Build history of the part. All positions in model axes, mm. A direction names the side the tool comes from. Round coordinates to 2 decimals unless told otherwise and drop trailing zeros. Write each loop counter-clockwise with the first axis right and the second up, starting at its lowest first coordinate (ties: lowest second). Pieces come first, ordered by that corner, then holes. Notation, with made-up numbers: (-29, 32.25) - (-1, 32.25) arc R15 cw to (-1, 60.25) - close; hole circle Ø8 at (-10.75, 44). An arc over 180 degrees is marked (long way). Answer as a JSON object with one key per item and string values. Group by question number.
Item 1: Which spindle directions (+Z, -Z, +X, -X, +Y, -Y) get a long thin tool onto all of the face, cutting with end or side? Do faces 1 (the cylindrical face through (14.117, -34.905, 19.399)), 2 (the flat face through (-15, -17, 26)), 3 (the cylindrical face through (-14.71, -34.9, 19.43)). Say none if no direction does.
Item 2: Flat gauge pins, fed straight in: pin 1 (8 mm diameter, centred on x = -34.5, y = -30.5, fed in from +Z); pin 2 (4 mm diameter, centred on y = -11.5, z = 15.5, fed in from +X); pin 3 (11 mm diameter, centred on y = -36, z = 12.5, fed in from +X). Where does each tip first touch, or does it go through?
Item 3: Two-plate mould, pull along Y, no slides. Class faces 4 (the flat face through (23, -17, 11)), 5 (the cylindrical face through (38.84, -27.63, 3.04)), 6 (the flat face through (14.688, -35, 13)): +Y half, -Y half, draft (parallel to the pull), parting line (faces both ways), or undercut.
Item 4: Slice it at B-B, the plane z = 40. List the corners of the cut face in (x, y), then the cut area to 3 significant figures.
Item 5: Slice it at A-A, the plane y = -9. Give the number of separate pieces and of enclosed holes in the cut face, then the cut area to 3 significant figures.
Item 6: Slice it at C-C, the plane x = -19. List the corners of the cut face in (y, z).
Item 7: Slice it at D-D, the plane z = 25. List the corners of the cut face in (x, y).
Item 8: Probe line 1 (X direction, y = -4, z = 11); line 2 (Z direction, x = 21, y = -11); line 3 (Y direction, x = 18, z = 19). List the from-to ranges inside material, lowest first. Write a range as from..to.
from build123d import *

# Parameters (mm, degrees)
F1_DEPTH  = 40
F14_R     = 4
F2_DEPTH  = 6
F3_R      = 4
F15_DEPTH = 6
F16_DEPTH = 14
F6_DEPTH  = 6
F17_DEPTH = 18
F18_DEPTH = 25
F8_DEPTH  = 20
F9_DEPTH  = 20
F10_DEPTH = 6
F12_DEPTH = 6
F13_DEPTH = 12


with BuildPart() as f1:
    # F0 (on Front) → F1 (new body)
    with BuildSketch(Plane.XZ):
        with BuildLine():
            Line((8.6878103536, 0), (45.6878103536, 0))
            Line((45.6878103536, 0), (45.6878103536, 6))
            Line((45.6878103536, 6), (16.6878103536, 6))
            ThreePointArc((16.6878103536, 6), (15.2735967912, 6.5857864376), (14.6878103536, 8))
            Line((14.6878103536, 8), (14.6878103536, 18))
            ThreePointArc((14.6878103536, 18), (14.102023916, 19.4142135624), (12.6878103536, 20))
            Line((12.6878103536, 20), (-13.3121896464, 20))
            ThreePointArc((-13.3121896464, 20), (-14.7264032088, 19.4142135624), (-15.3121896464, 18))
            Line((-15.3121896464, 18), (-15.3121896464, 6))
            Line((-15.3121896464, 6), (-46.3121896464, 6))
            Line((-46.3121896464, 6), (-46.3121896464, 0))
            Line((-46.3121896464, 0), (-9.3121896464, 0))
            Line((-9.3121896464, 0), (-9.3121896464, 12))
            ThreePointArc((-9.3121896464, 12), (-8.7264032088, 13.4142135624), (-7.3121896464, 14))
            Line((-7.3121896464, 14), (6.6878103536, 14))
            ThreePointArc((6.6878103536, 14), (8.102023916, 13.4142135624), (8.6878103536, 12))
            Line((8.6878103536, 12), (8.6878103536, 0))
        make_face()
    extrude(amount=F1_DEPTH)

    # F14 (on face) → F2 (cut)
    with BuildSketch(Plane.XY.offset(6)):
        with Locations((-37.3121896464, -31)):
            Circle(F14_R)
        with Locations((-37.3121896464, -9)):
            Circle(F14_R)
    extrude(amount=-F2_DEPTH, mode=Mode.SUBTRACT)

    # F3 (on face) → F15 (cut)
    with BuildSketch(Plane.XY.offset(6)):
        with Locations((36.6878103536, -31)):
            Circle(F3_R)
        with Locations((36.6878103536, -9)):
            Circle(F3_R)
    extrude(amount=-F15_DEPTH, mode=Mode.SUBTRACT)

    # F4 (on face) → F16 (join)
    with BuildSketch(Plane.XY.offset(20)):
        with BuildLine():
            Line((12.6878103536, -32.449899598), (12.6878103536, -7.550100402))
            ThreePointArc((12.6878103536, -7.550100402), (-0.3121896464, -2), (-13.3121896464, -7.550100402))
            Line((-13.3121896464, -7.550100402), (-13.3121896464, -32.449899598))
            ThreePointArc((-13.3121896464, -32.449899598), (-0.3121896464, -38), (12.6878103536, -32.449899598))
        make_face()
        with BuildLine():
            Line((-13.3121896464, -32.449899598), (-13.3121896464, -7.550100402))
            ThreePointArc((-13.3121896464, -7.550100402), (-18.3121896464, -20), (-13.3121896464, -32.449899598))
        make_face()
        with BuildLine():
            ThreePointArc((12.6878103536, -32.449899598), (16.3911034421, -26.7082039325), (17.6878103536, -20))
            ThreePointArc((17.6878103536, -20), (16.3911034421, -13.2917960675), (12.6878103536, -7.550100402))
            Line((12.6878103536, -7.550100402), (12.6878103536, -32.449899598))
        make_face()
    extrude(amount=-F16_DEPTH)

    # F5 (on face) → F6 (join)
    with BuildSketch(Plane.XY.offset(20)):
        with BuildLine():
            ThreePointArc((12.6878103536, -32.449899598), (16.3911034421, -26.7082039325), (17.6878103536, -20))
            ThreePointArc((17.6878103536, -20), (16.3911034421, -13.2917960675), (12.6878103536, -7.550100402))
            ThreePointArc((12.6878103536, -7.550100402), (-0.3121896464, -2), (-13.3121896464, -7.550100402))
            ThreePointArc((-13.3121896464, -7.550100402), (-18.3121896464, -20), (-13.3121896464, -32.449899598))
            ThreePointArc((-13.3121896464, -32.449899598), (-0.3121896464, -38), (12.6878103536, -32.449899598))
        make_face()
    extrude(amount=F6_DEPTH)

    # F7 (on face) → F17 (join)
    with BuildSketch(Plane.XY.offset(26)):
        with BuildLine():
            Line((-9.9985091191, -19.7734791318), (-14.9990061206, -19.7734791318))
            ThreePointArc((-14.9990061206, -19.7734791318), (-10.6674755741, -30.4915269508), (0, -34.9461504817))
            Line((0, -34.9461504817), (0, -29.9461504817))
            ThreePointArc((0, -29.9461504817), (-7.1318550707, -26.9559039189), (-9.9985091191, -19.7734791318))
        make_face()
        with BuildLine():
            ThreePointArc((15, -19.9461504817), (14.9997515281, -19.8598133766), (14.9990061206, -19.7734791318))
            Line((14.9990061206, -19.7734791318), (9.9985091191, -19.7734791318))
            ThreePointArc((9.9985091191, -19.7734791318), (9.9996272728, -19.8598115887), (10, -19.9461504817))
            ThreePointArc((10, -19.9461504817), (7.0710678119, -27.0172182936), (0, -29.9461504817))
            Line((0, -29.9461504817), (0, -34.9461504817))
            ThreePointArc((0, -34.9461504817), (10.6066017178, -30.5527521995), (15, -19.9461504817))
        make_face()
        with BuildLine():
            ThreePointArc((14.9990061206, -19.7734791318), (10.5453764691, -9.2786749076), (0, -4.9461504817))
            Line((0, -4.9461504817), (0, -9.9461504817))
            ThreePointArc((0, -9.9461504817), (7.0097534372, -12.814295411), (9.9985091191, -19.7734791318))
            Line((9.9985091191, -19.7734791318), (14.9990061206, -19.7734791318))
        make_face()
        with BuildLine():
            Line((0, -9.9461504817), (0, -4.9461504817))
            ThreePointArc((0, -4.9461504817), (-10.5453764691, -9.2786749076), (-14.9990061206, -19.7734791318))
            Line((-14.9990061206, -19.7734791318), (-9.9985091191, -19.7734791318))
            ThreePointArc((-9.9985091191, -19.7734791318), (-7.0097534372, -12.814295411), (0, -9.9461504817))
        make_face()
    extrude(amount=F17_DEPTH)

    # F18 (cut): a face of the model
    f18_faces = [f1.faces().sort_by_distance(p)[0] for p in [
        (0, -19.9461504817, 26),
    ]]
    extrude(f18_faces, amount=-F18_DEPTH, mode=Mode.SUBTRACT)

    # F19 (on face) → F8 (join)
    with BuildSketch(Plane.XY.offset(6)):
        with BuildLine():
            Line((36.6878103536, -23), (36.6878103536, -17))
            Line((36.6878103536, -17), (17.4360497029, -17))
            ThreePointArc((17.4360497029, -17), (17.6878103536, -20), (17.4360497029, -23))
            Line((17.4360497029, -23), (36.6878103536, -23))
        make_face()
    extrude(amount=F8_DEPTH)

    # F20 (on face) → F9 (join)
    with BuildSketch(Plane.XY.offset(6)):
        with BuildLine():
            Line((-18.0604289957, -17), (-37.3121896464, -17))
            Line((-37.3121896464, -17), (-37.3121896464, -23))
            Line((-37.3121896464, -23), (-18.0604289957, -23))
            ThreePointArc((-18.0604289957, -23), (-18.3121896464, -20), (-18.0604289957, -17))
        make_face()
    extrude(amount=F9_DEPTH)

    # F21 (on face) → F10 (cut)
    with BuildSketch(Plane.XZ.offset(23)):
        Polygon((17.4360497029, 26), (36.6878103536, 6), (36.6878103536, 26), align=None)
    extrude(amount=-F10_DEPTH, mode=Mode.SUBTRACT)

    # F11 (on face) → F12 (cut)
    with BuildSketch(Plane.XZ.offset(23)):
        Polygon((-37.3121896464, 26), (-37.3121896464, 6), (-18.0604289957, 26), align=None)
    extrude(amount=-F12_DEPTH, mode=Mode.SUBTRACT)

    # F13 (cut): faces of the model
    f13_faces = [f1.faces().sort_by_distance(p)[0] for p in [
        (-0.4565347665, -7.2840433998, 6),
        (-0.4547848435, -32.6635017138, 6),
        (-0.4565347665, -7.2840433998, 6),
        (-0.4547848435, -32.6635017138, 6),
    ]]
    extrude(f13_faces, amount=-F13_DEPTH, mode=Mode.SUBTRACT)


solid = f1.part
Geometry says:
{
 "1": {"face 1": "+Z, +X, -Y", "face 2": "+Z", "face 3": "+Z, -X, -Y"},
 "2": {"pin 1": "stops at z = 6", "pin 2": "stops at x = 16.47", "pin 3": "stops at x = 14.96"},
 "3": {"face 4": "+Y half", "face 5": "undercut", "face 6": "draft"},
 "4": {"outline": "circle Ø30 at (0, -19.95); hole circle Ø20 at (0, -19.95)", "area": "393 mm^2"},
 "5": {"separate pieces": "3", "enclosed holes": "0", "area": "1,090 mm^2"},
 "6": {"outline": "(-40, 0) - (0, 0) - (0, 6) - (-17, 6) - (-17, 25.02) - (-23, 25.02) - (-23, 6) - (-40, 6) - close"},
 "7": {"outline": "(-19.02, -23) - (-18.06, -23) arc R18 ccw to (17.44, -23) - (18.4, -23) - (18.4, -17) - (17.44, -17) arc R18 ccw to (-18.06, -17) - (-19.02, -17) - close; hole circle Ø20 at (0, -19.95)"},
 "8": {"line 1": "x = -15.31..-9.31, 8.69..14.69", "line 2": "z = 0..6", "line 3": "y = -23..-17"}
}
